```python
from build123d import *

# Parameters (mm, degrees)
SKETCH_1_W                       = 220
SKETCH_1_H                       = 135
LID_TOP_3MM_DEPTH                = 3
SKETCH_2_W                       = 216
SKETCH_2_H                       = 2
LID_RIM_BACK_DEPTH               = 12
SKETCH_3_W                       = 216
SKETCH_3_H                       = 2
LID_RIM_FRONT_DEPTH              = 12
SKETCH_4_W                       = 2
SKETCH_4_H                       = 135
LID_RIM_LEFT_DEPTH               = 12
SKETCH_5_W                       = 2
SKETCH_5_H                       = 135
LID_RIM_RIGHT_DEPTH              = 12
SKETCH_6_R                       = 1.8
LID_SCREW_CLEARANCE_1_DEPTH      = 16
SKETCH_7_R                       = 1.8
LID_SCREW_CLEARANCE_2_DEPTH      = 16
SKETCH_8_R                       = 1.8
LID_SCREW_CLEARANCE_3_DEPTH      = 16
SKETCH_9_R                       = 1.8
LID_SCREW_CLEARANCE_4_DEPTH      = 16
SKETCH_10_R                      = 9
OV5647_LENS_OPENING_D18_DEPTH    = 4
SKETCH_11_W                      = 34
SKETCH_11_H                      = 30
OV5647_SERVICE_CLEARANCE_DEPTH   = 4
SKETCH_12_R                      = 9.25
HC_SR04_ACOUSTIC_OPENING_1_DEPTH = 4
SKETCH_13_R                      = 9.25
HC_SR04_ACOUSTIC_OPENING_2_DEPTH = 4
SKETCH_14_W                      = 58
SKETCH_14_H                      = 34
HC_SR04_RECESS_DEPTH             = 1.2
SKETCH_15_W                      = 4
SKETCH_15_H                      = 24
VENT_SLOT_1_DEPTH                = 4
SKETCH_16_W                      = 4
SKETCH_16_H                      = 24
VENT_SLOT_2_DEPTH                = 4
SKETCH_17_W                      = 4
SKETCH_17_H                      = 24
VENT_SLOT_3_DEPTH                = 4
SKETCH_18_W                      = 4
SKETCH_18_H                      = 24
VENT_SLOT_4_DEPTH                = 4
SKETCH_19_W                      = 4
SKETCH_19_H                      = 24
VENT_SLOT_5_DEPTH                = 4
SKETCH_20_W                      = 4
SKETCH_20_H                      = 24
VENT_SLOT_6_DEPTH                = 4


with BuildPart() as part:
    # 草图1 → Lid_Top_3mm (new body)
    with BuildSketch(Plane(origin=(0, 0, 0), x_dir=(1, 0, 0), z_dir=(0, 1, 0))):
        Rectangle(SKETCH_1_W, SKETCH_1_H)
    extrude(amount=-LID_TOP_3MM_DEPTH)

    # 草图2 → Lid_Rim_Back (add)
    with BuildSketch(Plane(origin=(0, 0, 0), x_dir=(1, 0, 0), z_dir=(0, 1, 0))):
        with Locations((0, 66.5)):
            Rectangle(SKETCH_2_W, SKETCH_2_H)
    extrude(amount=-LID_RIM_BACK_DEPTH)

    # 草图3 → Lid_Rim_Front (add)
    with BuildSketch(Plane(origin=(0, 0, 0), x_dir=(1, 0, 0), z_dir=(0, 1, 0))):
        with Locations((0, -66.5)):
            Rectangle(SKETCH_3_W, SKETCH_3_H)
    extrude(amount=-LID_RIM_FRONT_DEPTH)

    # 草图4 → Lid_Rim_Left (add)
    with BuildSketch(Plane(origin=(0, 0, 0), x_dir=(1, 0, 0), z_dir=(0, 1, 0))):
        with Locations((-109, 0)):
            Rectangle(SKETCH_4_W, SKETCH_4_H)
    extrude(amount=-LID_RIM_LEFT_DEPTH)

    # 草图5 → Lid_Rim_Right (add)
    with BuildSketch(Plane(origin=(0, 0, 0), x_dir=(1, 0, 0), z_dir=(0, 1, 0))):
        with Locations((109, 0)):
            Rectangle(SKETCH_5_W, SKETCH_5_H)
    extrude(amount=-LID_RIM_RIGHT_DEPTH)

    # 草图6 → Lid_Screw_Clearance_1 (cut)
    with BuildSketch(Plane(origin=(0, 0, 0), x_dir=(1, 0, 0), z_dir=(0, 1, 0))):
        with Locations(Location((-100, -57, 0), (0, 0, 270))):
            Circle(SKETCH_6_R)
    extrude(amount=-LID_SCREW_CLEARANCE_1_DEPTH, mode=Mode.SUBTRACT)

    # 草图7 → Lid_Screw_Clearance_2 (cut)
    with BuildSketch(Plane(origin=(0, 0, 0), x_dir=(1, 0, 0), z_dir=(0, 1, 0))):
        with Locations(Location((100, -57, 0), (0, 0, 270))):
            Circle(SKETCH_7_R)
    extrude(amount=-LID_SCREW_CLEARANCE_2_DEPTH, mode=Mode.SUBTRACT)

    # 草图8 → Lid_Screw_Clearance_3 (cut)
    with BuildSketch(Plane(origin=(0, 0, 0), x_dir=(1, 0, 0), z_dir=(0, 1, 0))):
        with Locations(Location((-100, 57, 0), (0, 0, 270))):
            Circle(SKETCH_8_R)
    extrude(amount=-LID_SCREW_CLEARANCE_3_DEPTH, mode=Mode.SUBTRACT)

    # 草图9 → Lid_Screw_Clearance_4 (cut)
    with BuildSketch(Plane(origin=(0, 0, 0), x_dir=(1, 0, 0), z_dir=(0, 1, 0))):
        with Locations(Location((100, 57, 0), (0, 0, 270))):
            Circle(SKETCH_9_R)
    extrude(amount=-LID_SCREW_CLEARANCE_4_DEPTH, mode=Mode.SUBTRACT)

    # 草图10 → OV5647_Lens_Opening_D18 (cut)
    with BuildSketch(Plane(origin=(0, 0, 0), x_dir=(1, 0, 0), z_dir=(0, 1, 0))):
        with Locations(Location((-61, -34, 0), (0, 0, 270))):
            Circle(SKETCH_10_R)
    extrude(amount=-OV5647_LENS_OPENING_D18_DEPTH, mode=Mode.SUBTRACT)

    # 草图11 → OV5647_Service_Clearance (cut)
    with BuildSketch(Plane(origin=(0, 0, 0), x_dir=(1, 0, 0), z_dir=(0, 1, 0))):
        with Locations((-61, -34)):
            Rectangle(SKETCH_11_W, SKETCH_11_H)
    extrude(amount=-OV5647_SERVICE_CLEARANCE_DEPTH, mode=Mode.SUBTRACT)

    # 草图12 → HC_SR04_Acoustic_Opening_1 (cut)
    with BuildSketch(Plane(origin=(0, 0, 0), x_dir=(1, 0, 0), z_dir=(0, 1, 0))):
        with Locations(Location((46, -47, 0), (0, 0, 270))):
            Circle(SKETCH_12_R)
    extrude(amount=-HC_SR04_ACOUSTIC_OPENING_1_DEPTH, mode=Mode.SUBTRACT)

    # 草图13 → HC_SR04_Acoustic_Opening_2 (cut)
    with BuildSketch(Plane(origin=(0, 0, 0), x_dir=(1, 0, 0), z_dir=(0, 1, 0))):
        with Locations(Location((46, -21, 0), (0, 0, 270))):
            Circle(SKETCH_13_R)
    extrude(amount=-HC_SR04_ACOUSTIC_OPENING_2_DEPTH, mode=Mode.SUBTRACT)

    # 草图14 → HC_SR04_Recess (cut)
    with BuildSketch(Plane(origin=(0, 0, 0), x_dir=(1, 0, 0), z_dir=(0, 1, 0))):
        with Locations((46, -34)):
            Rectangle(SKETCH_14_W, SKETCH_14_H)
    extrude(amount=-HC_SR04_RECESS_DEPTH, mode=Mode.SUBTRACT)

    # 草图15 → Vent_Slot_1 (cut)
    with BuildSketch(Plane(origin=(0, 0, 0), x_dir=(1, 0, 0), z_dir=(0, 1, 0))):
        with Locations((-82, 42)):
            Rectangle(SKETCH_15_W, SKETCH_15_H)
    extrude(amount=-VENT_SLOT_1_DEPTH, mode=Mode.SUBTRACT)

    # 草图16 → Vent_Slot_2 (cut)
    with BuildSketch(Plane(origin=(0, 0, 0), x_dir=(1, 0, 0), z_dir=(0, 1, 0))):
        with Locations((-70, 42)):
            Rectangle(SKETCH_16_W, SKETCH_16_H)
    extrude(amount=-VENT_SLOT_2_DEPTH, mode=Mode.SUBTRACT)

    # 草图17 → Vent_Slot_3 (cut)
    with BuildSketch(Plane(origin=(0, 0, 0), x_dir=(1, 0, 0), z_dir=(0, 1, 0))):
        with Locations((-58, 42)):
            Rectangle(SKETCH_17_W, SKETCH_17_H)
    extrude(amount=-VENT_SLOT_3_DEPTH, mode=Mode.SUBTRACT)

    # 草图18 → Vent_Slot_4 (cut)
    with BuildSketch(Plane(origin=(0, 0, 0), x_dir=(1, 0, 0), z_dir=(0, 1, 0))):
        with Locations((-10, 42)):
            Rectangle(SKETCH_18_W, SKETCH_18_H)
    extrude(amount=-VENT_SLOT_4_DEPTH, mode=Mode.SUBTRACT)

    # 草图19 → Vent_Slot_5 (cut)
    with BuildSketch(Plane(origin=(0, 0, 0), x_dir=(1, 0, 0), z_dir=(0, 1, 0))):
        with Locations((2, 42)):
            Rectangle(SKETCH_19_W, SKETCH_19_H)
    extrude(amount=-VENT_SLOT_5_DEPTH, mode=Mode.SUBTRACT)

    # 草图20 → Vent_Slot_6 (cut)
    with BuildSketch(Plane(origin=(0, 0, 0), x_dir=(1, 0, 0), z_dir=(0, 1, 0))):
        with Locations((14, 42)):
            Rectangle(SKETCH_20_W, SKETCH_20_H)
    extrude(amount=-VENT_SLOT_6_DEPTH, mode=Mode.SUBTRACT)


solid = part.part
```
The listing builds one solid part. Answer for the finished solid, in the listing's coordinates (mm). A direction names the side the tool comes from. Round coordinates to 2 decimals unless told otherwise and drop trailing zeros. Write each loop counter-clockwise with the first axis right and the second up, starting at its lowest first coordinate (ties: lowest second). Pieces come first, ordered by that corner, then holes. Notation, with made-up numbers: (60.5, 47.5) -> (75.5, 47.5) arc R36 ccw to (75.5, 84.5) -> close; hole circle Ø7 at (10, 62.25). An arc over 180 degrees is marked (long way). Use CSV: the item, a comma, the result in double quotes. Start each with the question number.
(1) Which of the six approach directions +Z, -Z, +X, -X, +Y, -Y give full straight-line access (tool end or side, diameter ignored) to faces 4 (the face through (108, -7, 1)), 5 (the face through (46, -1.2, 34)), 6 (the face through (110, -6, 1))?
(2) Section A-A on z = 24 is taken. Give the vertices of the cut face in (x, y), then the cut area to 3 significant figures.
(3) The mould has two halves that part along Z. Classify faces 1 (the face through (-2, -6, 67.5)), 2 (the face through (-110, -6, 1)), 3 (the face through (-108, -7, 1)): released by +Z, released by -Z, zero draft, split by the parting line, or undercut.
(4) Section C-C on x = 46 is taken. Give the vertices of the cut face in (y, z), then the cut area to 3 significant figures.
(5) Each of these flat-tipped pins is pushed along its axis until it touches: pin 1 (2 mm diameter, centred on x = -100, z = -57, fed in from -Y); pin 2 (17 mm diameter, centred on x = 52, z = 30.5, fed in from +Y). Where does it stop, or does it pass through?
(6) Consider L1, parallel to X at y = -2.15, z = -57; L2, parallel to Z at x = 46, y = -2.15; L3, parallel to X at y = -2.2, z = 21. Determine where each line is inside the solid, lowest interval first. Write a range as from..to.
(7) Section D-D on z = -22.5 is taken. Give the vertices of the cut face in (x, y), then the cut area to 3 significant figures.
(8) Section B-B on y = -7.5 is taken. Give the vertices of the cut face in (x, z).
A:
1,face 4,"-Y"
1,face 5,"+Y"
1,face 6,"+Z, -Z, +X, +Y, -Y"
2,outline,"(-110, -12) -> (-108, -12) -> (-108, -3) -> (-78, -3) -> (-78, 0) -> (-110, 0) -> close; (-44, -3) -> (37.25, -3) -> (37.25, -1.2) -> (17, -1.2) -> (17, 0) -> (-44, 0) -> close; (54.75, -3) -> (108, -3) -> (108, -12) -> (110, -12) -> (110, 0) -> (75, 0) -> (75, -1.2) -> (54.75, -1.2) -> close"
2,area,"493 mm²"
3,face 1,"released by +Z"
3,face 2,"zero draft"
3,face 3,"undercut"
4,outline,"(-12, -67.5) -> (0, -67.5) -> (0, 11.75) -> (-3, 11.75) -> (-3, -65.5) -> (-12, -65.5) -> close; (-12, 65.5) -> (-3, 65.5) -> (-3, 56.25) -> (0, 56.25) -> (0, 67.5) -> (-12, 67.5) -> close; (-3, 30.25) -> (-1.2, 30.25) -> (-1.2, 37.75) -> (-3, 37.75) -> close"
4,area,"321 mm²"
5,pin 1,"passes through"
5,pin 2,"stops at y = -1.2"
6,L1,"x = -110..-101.8, -98.2..98.2, 101.8..110"
6,L2,"z = -67.5..11.75, 30.25..37.75, 56.25..67.5"
6,L3,"x = -110..-78, -44..36.75, 55.25..110"
7,outline,"(-110, -12) -> (-108, -12) -> (-108, -3) -> (108, -3) -> (108, -12) -> (110, -12) -> (110, 0) -> (-110, 0) -> close"
7,area,"696 mm²"
8,outline,"(-110, -67.5) -> (110, -67.5) -> (110, 67.5) -> (-110, 67.5) -> close; hole (-108, -65.5) -> (108, -65.5) -> (108, 65.5) -> (-108, 65.5) -> close"
